Check sheet for the modelled part. Datum: model origin and axes. Units: mm. A direction names the side the tool comes from. Round coordinates to 2 decimals unless told otherwise and drop trailing zeros. Order: outer loops, then holes, each group sorted by start corner. A loop starts at its lowest first (then second) coordinate and runs counter-clockwise, first axis right, second up. Notation, with made-up numbers: M 21.5,37.5 L 55.5,37.5 A20 ccw 55.5,50.5 Z; hole C -5.5,20 d10. An arc over 180 degrees is marked long. One line per item, written item: value. Start each with the question number.
(1) Cross-section at A-A, the plane z = 0. Enter the section's corners in (x, y).
(2) Depth check by flat-ended pin: pin 1 Ø6 at (x, y) = (8, 4.5) entering from -Z; pin 2 Ø5 at (x, z) = (-0.5, -5) entering from +Y; pin 3 Ø3 at (y, z) = (-9, 37.5) entering from +X. Enter the tip coordinate at first touch or a pass-through.
(3) Cross-section at D-D, the plane z = 34. Enter the section's corners in (x, y), and give its area (3 significant figures).
(4) Cross-section at B-B, the plane x = 0. Count the separate pieces of the cut face and the enclosed holes in it, and give its area (3 significant figures).
(5) Access from +Z, -Z, +X, -X, +Y, -Y to the whole of each face (thin tool, end or side, straight path). Record for faces 4 (the face through (0.064, -2.724, 51.922)), 5 (the face through (-16.498, 11.77, -14.665)), 6 (the face through (-18.806, -2.724, 21.244)).
(6) Release check for a two-part mould opening along X. For faces 1 (the face through (-5, -22.7, 2)), 2 (the face through (-3, -18.7, 3)), 3 (the face through (-9.85, -2.72, 41)) record: released by +X, released by -X, zero draft, split by the parting line, or undercut.
(7) Thickness scan on L1, parallel to X at y = -1, z = 0; L2, parallel to Z at x = -7, y = 14; L3, parallel to Z at x = 13.5, y = 10. Record the ranges inside material, lowest first.
from build123d import *

# Parameters (mm, degrees)
SKETCH1_W                       = 39.4
SKETCH1_H                       = 38.1
BOSS_EXTRUDE1_DEPTH             = 19.05
SKETCH1_3_W                     = 4
SKETCH1_3_H                     = 3.96875
CUT_REVOLVE2_OUTLINE_W          = 12.7
CUT_REVOLVE2_OUTLINE_H          = 16.276210188
SKETCH1_5_W                     = 1
SKETCH1_5_H                     = 1.5875
FILLET2_R                       = 0.1
SKETCH2_R                       = 2.413
CUT_EXTRUDE1_DEPTH              = 10
EXTRUDE_THIN1_REACH             = 37.229
EXTRUDE_THIN1_DIRECTION_2_REACH = 37.229
FILLET5_R                       = 4


# Read off the part's stored shape, not the designer's step: Cut-Revolve2
with BuildPart() as part:
    # Sketch1 → Boss-Extrude1 (new, symmetric)
    with BuildSketch(Plane.YZ):
        with Locations((-3, 0)):
            Rectangle(SKETCH1_W, SKETCH1_H)
    extrude(amount=BOSS_EXTRUDE1_DEPTH, both=True)

    # Sketch1_3 → Cut-Revolve1 (revolve, cut)
    with BuildSketch(Plane.YZ):
        Polygon((12.7, 0), (16.7, 0), (16.7, 13), (-18.7, 13), (-18.7, 3.96875), (-18.7, 0), (-12.7, 0), (0, 0), align=None)
        with Locations((-20.7, 1.984375)):
            Rectangle(SKETCH1_3_W, SKETCH1_3_H)
    revolve(axis=Axis((0, 16.7, 0), (0, -1, 0)), mode=Mode.SUBTRACT)

    # Cut-Revolve2 outline → Cut-Revolve2 (revolve, cut)
    with BuildSketch(Plane.XZ):
        with Locations((6.35, -10.911894906)):
            Rectangle(CUT_REVOLVE2_OUTLINE_W, CUT_REVOLVE2_OUTLINE_H)
    revolve(axis=Axis((0, 0, 0), (0, 0, 1)), mode=Mode.SUBTRACT)

    # Sketch1_5 → Cut-Revolve3 (revolve, cut)
    with BuildSketch(Plane.YZ):
        with Locations((16.2, 14.79375)):
            Rectangle(SKETCH1_5_W, SKETCH1_5_H)
    revolve(axis=Axis((0, 16.7, 0), (0, -1, 0)), mode=Mode.SUBTRACT)

    # Fillet2
    fillet2_edges = [part.edges().sort_by_distance(p)[0] for p in [
        (0, 15.7, -15.5875),
        (0, 15.7, -14),
        (0, 16.7, -14),
        (0, 16.7, -15.5875),
    ]]
    fillet(fillet2_edges, radius=FILLET2_R)

    # Sketch2 → Cut-Extrude1 (cut)
    with BuildSketch(Plane(origin=(0, 16.7, 0), x_dir=(-1, 0, 0), z_dir=(0, 1, 0))):
        with Locations(Location((-14.142135624, 14.142135624, 0), (0, 0, 90))):
            Circle(SKETCH2_R)
        with Locations(Location((14.142135624, 14.142135624, 0), (0, 0, 90))):
            Circle(SKETCH2_R)
        with Locations(Location((14.142135624, -14.142135624, 0), (0, 0, 90))):
            Circle(SKETCH2_R)
        with Locations(Location((-14.142135624, -14.142135624, 0), (0, 0, 90))):
            Circle(SKETCH2_R)
    extrude(amount=-CUT_EXTRUDE1_DEPTH, mode=Mode.SUBTRACT)

    # Extrude-Thin1: up to this face of the body (flat: up to its plane)
    extrude_thin1_end = Plane(part.part.faces().sort_by_distance((-18.511184633, 16.7, 0))[0])
    # Sketch3 → Extrude-Thin1 (add, up to the picked face)
    with BuildSketch(Plane(origin=(0, 0, 0), x_dir=(-1, 0, 0), z_dir=(0, 1, 0)), mode=Mode.PRIVATE) as extrude_thin1_sk1:
        with BuildLine():
            ThreePointArc((-19.05, 19.05), (-18.812960071, 21.214396139), (-18.11307787, 23.276182617))
            Line((-18.11307787, 23.276182617), (-1.812615574, 58.232636819))
            ThreePointArc((-1.812615574, 58.232636819), (0, 59.387400296), (1.812615574, 58.232636819))
            Line((1.812615574, 58.232636819), (18.11307787, 23.276182617))
            ThreePointArc((18.11307787, 23.276182617), (18.812960071, 21.214396139), (19.05, 19.05))
            Line((19.05, 19.05), (17.05, 19.05))
            ThreePointArc((17.05, 19.05), (16.860368057, 20.781516912), (16.300462296, 22.430946094))
            Line((16.300462296, 22.430946094), (0, 57.387400296))
            Line((0, 57.387400296), (-16.300462296, 22.430946094))
            ThreePointArc((-16.300462296, 22.430946094), (-16.860368057, 20.781516912), (-17.05, 19.05))
            Line((-17.05, 19.05), (-19.05, 19.05))
        make_face()
    extrude_thin1_tool1 = split(extrude(extrude_thin1_sk1.sketch, amount=EXTRUDE_THIN1_REACH, mode=Mode.PRIVATE), bisect_by=extrude_thin1_end, keep=Keep.BOTH, mode=Mode.PRIVATE)
    add(extrude_thin1_tool1.solids().sort_by(Axis((18.271251, 0, 21.094302), (0, 1, 0)))[0])

    # Extrude-Thin1 direction 2: up to this face of the body (flat: up to its plane)
    extrude_thin1_direction_2_end = Plane(part.part.faces().sort_by_distance((0, -22.7, 18.511184633))[0])
    # Sketch3 → Extrude-Thin1 direction 2 (add, up to the picked face)
    with BuildSketch(Plane(origin=(0, 0, 0), x_dir=(-1, 0, 0), z_dir=(0, 1, 0)), mode=Mode.PRIVATE) as extrude_thin1_direction_2_sk1:
        with BuildLine():
            ThreePointArc((-19.05, 19.05), (-18.812960071, 21.214396139), (-18.11307787, 23.276182617))
            Line((-18.11307787, 23.276182617), (-1.812615574, 58.232636819))
            ThreePointArc((-1.812615574, 58.232636819), (0, 59.387400296), (1.812615574, 58.232636819))
            Line((1.812615574, 58.232636819), (18.11307787, 23.276182617))
            ThreePointArc((18.11307787, 23.276182617), (18.812960071, 21.214396139), (19.05, 19.05))
            Line((19.05, 19.05), (17.05, 19.05))
            ThreePointArc((17.05, 19.05), (16.860368057, 20.781516912), (16.300462296, 22.430946094))
            Line((16.300462296, 22.430946094), (0, 57.387400296))
            Line((0, 57.387400296), (-16.300462296, 22.430946094))
            ThreePointArc((-16.300462296, 22.430946094), (-16.860368057, 20.781516912), (-17.05, 19.05))
            Line((-17.05, 19.05), (-19.05, 19.05))
        make_face()
    extrude_thin1_direction_2_tool1 = split(extrude(extrude_thin1_direction_2_sk1.sketch, amount=-EXTRUDE_THIN1_DIRECTION_2_REACH, mode=Mode.PRIVATE), bisect_by=extrude_thin1_direction_2_end, keep=Keep.BOTH, mode=Mode.PRIVATE)
    add(extrude_thin1_direction_2_tool1.solids().sort_by(Axis((18.271251, 0, 21.094302), (0, -1, 0)))[0])

    # Fillet5
    fillet5_edges = [part.edges().sort_by_distance(p)[0] for p in [
        (0, -3, 57.387400296),
        (17.05, -3, 19.05),
        (-17.05, -3, 19.05),
    ]]
    fillet(fillet5_edges, radius=FILLET5_R)


solid = part.part
Values found:
1. outline: M -19.05,-22.7 L -3.97,-22.7 L -3.97,-18.7 L -13,-18.7 L -13,16.7 L -13.9,16.7 A0.1 ccw -14,16.6 L -14,15.8 A0.1 cw -14.1,15.7 L -15.49,15.7 A0.1 cw -15.59,15.8 L -15.59,16.6 A0.1 ccw -15.69,16.7 L -19.05,16.7 Z; M 3.97,-22.7 L 19.05,-22.7 L 19.05,16.7 L 15.69,16.7 A0.1 ccw 15.59,16.6 L 15.59,15.8 A0.1 cw 15.49,15.7 L 14.1,15.7 A0.1 cw 14,15.8 L 14,16.6 A0.1 ccw 13.9,16.7 L 13,16.7 L 13,-18.7 L 3.97,-18.7 Z
2. pin 1: z = 6.93
2. pin 2: y = -18.7
2. pin 3: x = 12.18
3. outline: M -13.11,-22.7 L -10.91,-22.7 L -10.91,16.7 L -13.11,16.7 Z; M 10.91,-22.7 L 13.11,-22.7 L 13.11,16.7 L 10.91,16.7 Z
3. area: 174 mm^2
4. separate pieces: 4
4. enclosed holes: 0
4. area: 686 mm^2
5. face 4: +Y, -Y
5. face 5: +Y
5. face 6: +Z, -X, +Y, -Y
6. face 1: zero draft
6. face 2: undercut
6. face 3: released by -X
7. L1: -19.05 to -13, 13 to 19.05
7. L2: -19.05 to -10.95, 10.95 to 19.05, 42.38 to 47.11
7. L3: -19.05 to -16.47, -11.82 to 11.82, 16.47 to 19.53, 28.44 to 33.17
